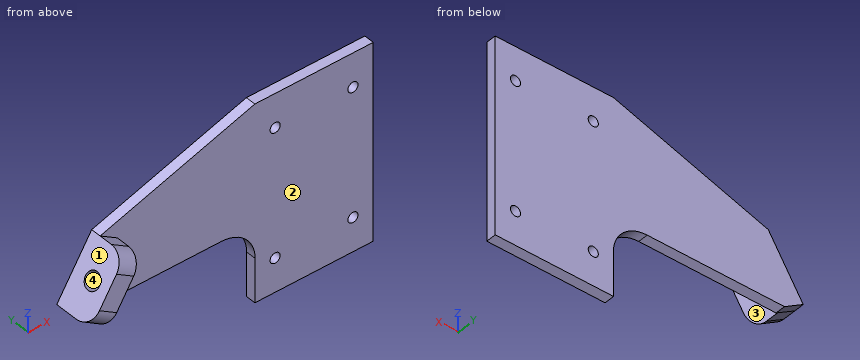
```python
from build123d import *

# Parameters (mm, degrees)
F1_DEPTH = 3
F4_DEPTH = 9
F5_R     = 5
F6_D     = 3
F8_D     = 5
F9_R     = 10


with BuildPart() as f1:
    # F0 (on Front) → F1 (new body)
    with BuildSketch(Plane.XZ):
        Polygon((-35, 0), (0, 0), (0, 58), (-35, 58), (-80.7513064809, 43), (-91.0847321335, 26.4630621249), (-85.5426742387, 23), (-34.875433892, 23), align=None)
    extrude(amount=-F1_DEPTH)

    # F3 (on face) → F4 (join)
    with BuildSketch(Plane.XZ):
        Polygon((-75.663017904, 39.8204844146), (-80.7513064809, 43), (-91.0847321335, 26.4630621249), (-85.9964435565, 23.2835465396), align=None)
    extrude(amount=F4_DEPTH)

    # F5
    f5_edges = [f1.edges().sort_by_distance(p)[0] for p in [
        (-78.207162, -9, 41.410242),
        (-88.540588, -9, 24.873304),
    ]]
    fillet(f5_edges, radius=F5_R)

    # F6 (through all)
    with Locations(Plane.XZ):
        with Locations((-29, 48), (-6, 48), (-6, 10), (-29, 10)):
            Hole(F6_D / 2)

    # F8 (through all)
    with Locations(Plane(origin=(-77.3992466493, 0, 48.364417092), x_dir=(0, -1, 0), z_dir=(-0.8480480962, 0, 0.5299192642))):
        with Locations((3.5, -16.0756047815)):
            Hole(F8_D / 2)

    # F9
    f9_edges = [f1.edges().sort_by_distance(p)[0] for p in [
        (-34.875434, 1.5, 23),
    ]]
    fillet(f9_edges, radius=F9_R)


solid = f1.part
```
The listing builds one solid part. Answer for the finished solid, in the listing's coordinates (mm). Face numbers are marked on the shaded views. Give positions to 0.01 mm unless a question says otherwise; leave off trailing zeros. Order: outer loops, then holes, each group sorted by start corner. A loop starts at its lowest first (then second) coordinate and runs counter-clockwise, first axis right, second up. Notation, with made-up numbers: (25.5, -7.5) - (32.5, -7.5) arc R29 cw to (32.5, 14.5) - close; hole circle Ø4 at (-34, -11.5). An arc over 180 degrees is marked (long way). Use one line per item in the form item = value. Start each with the question number.
(1) The mould has two halves that part along X. Classify the marked faces 1, 2, 3 and 4: released by +X, released by -X, zero draft, split by the parting line, or undercut.
(2) A cutting plane is placed at A-A, the plane x = -6. Write down the section's boundary in (y, z), then the cut area to 3 significant figures.
(3) Consider line 1 (Z direction, x = -6, y = 1.8); line 2 (Y direction, x = -3.5, z = 9); line 3 (Z direction, x = -39.5, y = 1.5). Determine where each line is inside the solid, lowest interval first. Write a range as from..to.
(4) A cutting plane is placed at C-C, the plane z = 48. Write down the section's boundary in (x, y).
(5) Flat-ended cylindrical pins translate along their axes: pin 1 Ø0.9 at (x, y) = (-65.5, 2) entering from -Z; pin 2 Ø5 at (y, z) = (-4, 41) entering from -X; pin 3 Ø2.5 at (x, z) = (-6, 48) entering from +Y; pin 4 Ø10 at (x, z) = (-33.5, 14) entering from -Y. Find the tip coordinate at first contact, or state that the pin passes through.
(6) A cutting plane is placed at D-D, the plane y = -7.75. Write down the section's boundary in (x, z).
(7) A cutting plane is placed at B-B, the plane y = -3. Write down the section's boundary in (x, z), then the cut area to 3 significant figures.
Ans:
q1.face_1 = released by -X
q1.face_2 = zero draft
q1.face_3 = released by +X
q1.face_4 = undercut
q2.outline = (0, 0) - (3, 0) - (3, 8.5) - (0, 8.5) - close; (0, 11.5) - (3, 11.5) - (3, 46.5) - (0, 46.5) - close; (0, 49.5) - (3, 49.5) - (3, 58) - (0, 58) - close
q2.area = 156 mm^2
q3.line_1 = 0..8.5, 11.5..46.5, 49.5..58
q3.line_2 = 0..3
q3.line_3 = 21.4..56.52
q4.outline = (-65.5, 0) - (-30.5, 0) - (-30.5, 3) - (-65.5, 3) - close; (-27.5, 0) - (-7.5, 0) - (-7.5, 3) - (-27.5, 3) - close; (-4.5, 0) - (0, 0) - (0, 3) - (-4.5, 3) - close
q5.pin_1 = 23
q5.pin_2 = -83.56
q5.pin_3 = through
q5.pin_4 = 0
q6.outline = (-90.19, 27.9) - (-85.1, 24.72) - (-76.56, 38.38) - (-81.65, 41.56) - close
q7.outline = (-91.08, 26.46) - (-86, 23.28) - (-82.13, 29.47) - (-87.22, 32.65) - close; (-84.62, 36.81) - (-79.53, 33.63) - (-75.66, 39.82) - (-80.75, 43) - close
q7.area = 87.6 mm^2
